Can you work these out from the model? Positions are in its coordinate system, mm. Coordinates: 2 decimals unless noted, no trailing zeros. Order: outer loops, then holes, each group sorted by start corner. A loop starts at its lowest first (then second) coordinate and runs counter-clockwise, first axis right, second up. Notation, with made-up numbers: (-35, -36) -> (4, -36) arc R14 cw to (4, -9) -> close; hole circle Ø8 at (83, 85.25). An arc over 180 degrees is marked (long way). Answer in a Markdown table with one row per item. Add a question column.
1. If I drill on line 1 along Y through (x, z) = (17.5, 2); line 2 along X through (y, z) = (-31.5, 1.45); line 3 along X through (y, z) = (-31, 2.6), over which ranges is the centre line in solid material (lowest first)? Write a range as [from, to].
2. Imagine slicing it at B-B on x = 17.5. Write out the boundary of the cut face in (y, z), plus the area to 3 significant figures.
3. Imagine slicing it at A-A on y = -31.5. Write out the boundary of the cut face in (x, z), plus the area to 3 significant figures.
4. Will these pins go through, and if not, where does the flat tip stop? pin 1 (1.5 mm diameter, centred on x = 21.5, y = -18, fed in from -Z); pin 2 (4.5 mm diameter, centred on x = 17.5, y = -31.5, fed in from -Z).
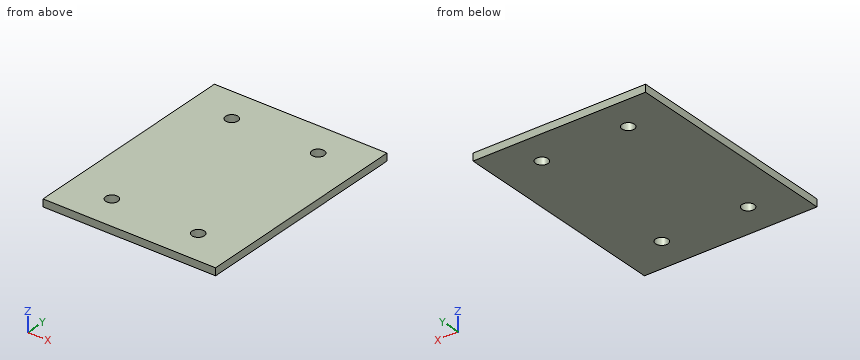
from build123d import *

# Parameters (mm, degrees)
SKETCH1_W           = 70
SKETCH1_H           = 90
BOSS_EXTRUDE1_DEPTH = 3
SKETCH2_R           = 2.5
CUT_EXTRUDE1_DEPTH  = 58.087651905


with BuildPart() as part:
    # Sketch1 → Boss-Extrude1 (new body)
    with BuildSketch(Plane.XY):
        Rectangle(SKETCH1_W, SKETCH1_H)
    extrude(amount=BOSS_EXTRUDE1_DEPTH)

    # Sketch2 → Cut-Extrude1 (cut, through all)
    with BuildSketch(Plane.XY.offset(3)):
        with Locations((-17.5, 31.5)):
            Circle(SKETCH2_R)
        with Locations((17.5, 31.5)):
            Circle(SKETCH2_R)
    cut_extrude1 = extrude(amount=-CUT_EXTRUDE1_DEPTH, mode=Mode.SUBTRACT)

    # Mirror1: Cut-Extrude1 across plane
    add(cut_extrude1.mirror(Plane.ZX), mode=Mode.SUBTRACT)


solid = part.part
Answers follow:
| question | item | result |
|---|---|---|
| 1 | line 1 | y = [-45, -34], [-29, 29], [34, 45] |
| 1 | line 2 | x = [-35, -20], [-15, 15], [20, 35] |
| 1 | line 3 | x = [-35, -19.95], [-15.05, 15.05], [19.95, 35] |
| 2 | outline | (-45, 0) -> (-34, 0) -> (-34, 3) -> (-45, 3) -> close; (-29, 0) -> (29, 0) -> (29, 3) -> (-29, 3) -> close; (34, 0) -> (45, 0) -> (45, 3) -> (34, 3) -> close |
| 2 | area | 240 mm² |
| 3 | outline | (-35, 0) -> (-20, 0) -> (-20, 3) -> (-35, 3) -> close; (-15, 0) -> (15, 0) -> (15, 3) -> (-15, 3) -> close; (20, 0) -> (35, 0) -> (35, 3) -> (20, 3) -> close |
| 3 | area | 180 mm² |
| 4 | pin 1 | stops at z = 0 |
| 4 | pin 2 | passes through |
